```python
from build123d import *

# Parameters (mm, degrees)
SKETCH2_W                 = 76.2
SKETCH2_H                 = 45.72
BOSS_EXTRUDE3_DEPTH       = 11.684
SKETCH6_R                 = 1.7272
CUT_EXTRUDE2_DEPTH        = 90.628534831
SKETCH7_R                 = 1.7272
CUT_EXTRUDE3_DEPTH        = 90.628534831
SKETCH8_R                 = 1.7272
CUT_EXTRUDE4_DEPTH        = 90.628534831
SKETCH9_R                 = 1.397
CUT_EXTRUDE5_DEPTH        = 15.24
F_4_40_TAPPED_HOLE1_D     = 2.2606
F_4_40_TAPPED_HOLE1_DEPTH = 7.62
F_4_40_TAPPED_HOLE1_TIP   = 0.679152758
F_8_32_TAPPED_HOLE1_D     = 3.4544
F_8_32_TAPPED_HOLE1_DEPTH = 12.446
F_8_32_TAPPED_HOLE1_TIP   = 1.037806461
F_8_32_TAPPED_HOLE2_D     = 3.4544
F_8_32_TAPPED_HOLE2_DEPTH = 12.446
F_8_32_TAPPED_HOLE2_TIP   = 1.037806461
FILLET1_R                 = 2.54


with BuildPart() as part:
    # Sketch2 → Boss-Extrude3 (new body)
    with BuildSketch(Plane(origin=(0, 0, 0), x_dir=(1, 0, 0), z_dir=(0, 1, 0))):
        with Locations((38.1, -22.86)):
            Rectangle(SKETCH2_W, SKETCH2_H)
    extrude(amount=BOSS_EXTRUDE3_DEPTH)

    # Sketch6 → Cut-Extrude2 (cut, through all)
    with BuildSketch(Plane(origin=(0, 11.684, 0), x_dir=(1, 0, 0), z_dir=(0, 1, 0))):
        with Locations(Location((7.62, -22.86, 0), (0, 0, 270))):
            Circle(SKETCH6_R)
    extrude(amount=-CUT_EXTRUDE2_DEPTH, mode=Mode.SUBTRACT)

    # Sketch7 → Cut-Extrude3 (cut, through all)
    with BuildSketch(Plane(origin=(0, 11.684, 0), x_dir=(1, 0, 0), z_dir=(0, 1, 0))):
        with Locations(Location((69.85, -8.89, 0), (0, 0, 270))):
            Circle(SKETCH7_R)
    extrude(amount=-CUT_EXTRUDE3_DEPTH, mode=Mode.SUBTRACT)

    # Sketch8 → Cut-Extrude4 (cut, through all)
    with BuildSketch(Plane(origin=(0, 11.684, 0), x_dir=(1, 0, 0), z_dir=(0, 1, 0))):
        with Locations(Location((69.85, -36.83, 0), (0, 0, 270))):
            Circle(SKETCH8_R)
    extrude(amount=-CUT_EXTRUDE4_DEPTH, mode=Mode.SUBTRACT)

    # Sketch9 → Cut-Extrude5 (cut)
    with BuildSketch(Plane.ZY):
        with Locations((27.94, 9.017)):
            Circle(SKETCH9_R)
    extrude(amount=-CUT_EXTRUDE5_DEPTH, mode=Mode.SUBTRACT)

    # #4-40 Tapped Hole1
    with Locations(Plane(origin=(0, 0, 0), x_dir=(-1, 0, 0), z_dir=(0, -1, 0))):
        with Locations((-3.175, -3.5052), (-3.175, -37.1602), (-14.605, -3.5052), (-14.605, -37.1602)):
            Hole(F_4_40_TAPPED_HOLE1_D / 2, depth=F_4_40_TAPPED_HOLE1_DEPTH)
            with Locations((0, 0, -(F_4_40_TAPPED_HOLE1_DEPTH + F_4_40_TAPPED_HOLE1_TIP / 2))):  # 118° drill point
                Cone(0, F_4_40_TAPPED_HOLE1_D / 2, F_4_40_TAPPED_HOLE1_TIP, mode=Mode.SUBTRACT)

    # #8-32 Tapped Hole1
    with Locations(Plane(origin=(70.866, 0, 20.574), x_dir=(0, 0, -1), z_dir=(0, -1, 0))):
        with Locations((0, 0)):
            Hole(F_8_32_TAPPED_HOLE1_D / 2, depth=F_8_32_TAPPED_HOLE1_DEPTH)
            with Locations((0, 0, -(F_8_32_TAPPED_HOLE1_DEPTH + F_8_32_TAPPED_HOLE1_TIP / 2))):  # 118° drill point
                Cone(0, F_8_32_TAPPED_HOLE1_D / 2, F_8_32_TAPPED_HOLE1_TIP, mode=Mode.SUBTRACT)

    # #8-32 Tapped Hole2
    with Locations(Plane(origin=(35.814, 0, 16.002), x_dir=(0, 0, -1), z_dir=(0, -1, 0))):
        with Locations((0, 0)):
            Hole(F_8_32_TAPPED_HOLE2_D / 2, depth=F_8_32_TAPPED_HOLE2_DEPTH)
            with Locations((0, 0, -(F_8_32_TAPPED_HOLE2_DEPTH + F_8_32_TAPPED_HOLE2_TIP / 2))):  # 118° drill point
                Cone(0, F_8_32_TAPPED_HOLE2_D / 2, F_8_32_TAPPED_HOLE2_TIP, mode=Mode.SUBTRACT)

    # Fillet1
    fillet1_edges = [part.edges().sort_by_distance(p)[0] for p in [
        (0, 5.842, 0),
        (76.2, 5.842, 0),
        (76.2, 5.842, 45.72),
        (0, 5.842, 45.72),
    ]]
    fillet(fillet1_edges, radius=FILLET1_R)


solid = part.part
```
Source: CAD feature listing. Evaluate the final solid. Frame: model axes, mm. A direction names the side the tool comes from. Coordinates: 2 decimals unless noted, no trailing zeros. Loops run counter-clockwise (first coordinate to the right, second up) from the corner with the lowest first, then second, coordinate; pieces in that order, holes last. Notation, with made-up numbers: M 7.25,-2.5 L 43.25,-2.5 A18 cw 43.25,10.5 Z; hole C -26,-9 d3. An arc over 180 degrees is marked long. Use CSV: the item, a comma, the result in double quotes.
(1) Draft query along Y for faces 4 (the face through (7.513, 10.195, 28.691)), 5 (the face through (14.36, 3.863, 38.264)), 6 (the face through (38, 0, 23)). Return one class per face: pulls with the +Y half, pulls with the -Y half, needs draft (parallel to the pull), parting line crosses it, or undercut.
Answers follow:
face 4,"undercut"
face 5,"needs draft"
face 6,"pulls with the -Y half"
(2) Line query: line 1 (X direction, y = 3.75, z = 20.5); line 2 (Y direction, x = 8, z = 27.94); line 3 (X direction, y = 7, z = 38). Output: solid intervals per line, ascending. Write a range as [from, to].
Answers follow:
line 1,"[0, 69.14], [72.59, 76.2]"
line 2,"[0, 7.62], [10.41, 11.68]"
line 3,"[0, 2.42], [3.93, 13.85], [15.36, 68.58], [71.12, 76.2]"
(3) Contact query for flat-ended pins moving along their axis: pin 1 (0.8 mm diameter, centred on y = 8.5, z = 27.5, fed in from -X); pin 2 (1.8 mm diameter, centred on x = 14.6, z = 3.51, fed in from -Y). Output: stop coordinate, or through.
Answers follow:
pin 1,"x = 15.24"
pin 2,"y = 7.75"
(4) Cut plane B-B on y = 1.5. Give the number of separate pieces and of enclosed holes in the cut face, and give its area (3 significant figures).
Answers follow:
separate pieces,"1"
enclosed holes,"9"
area,"3,420 mm²"
(5) Cut plane A-A on z = 27.94. Return loops of the section in (x, y).
Answers follow:
outline,"M 0,0 L 76.2,0 L 76.2,11.68 L 0,11.68 L 0,10.41 L 15.24,10.41 L 15.24,7.62 L 0,7.62 Z"
(6) Reachability of faces 1 (the face through (15.24, 9, 28)), 2 (the face through (0.724, 5.924, 0.764)), 3 (the face through (2.278, 3.863, 4.193)) from +Z, -Z, +X, -X, +Y, -Y: full face, straight path, thin tool, end or side. Return the list, or none.
Answers follow:
face 1,"-X"
face 2,"-Z, -X, +Y, -Y"
face 3,"-Y"
